Geometry check sheet. Reference: the model listing, model coordinates, mm. A direction names the side the tool comes from. Round coordinates to 2 decimals unless told otherwise and drop trailing zeros. Order: outer loops, then holes, each group sorted by start corner. A loop starts at its lowest first (then second) coordinate and runs counter-clockwise, first axis right, second up.
```python
from build123d import *

# Parameters (mm, degrees)
EXTRUDE_1_DEPTH          = 2
EXTRUDE_1_2_DEPTH        = 2
EXTRUDE_3_DEPTH          = 33.5
EXTRUDE_3_DEPTH_BACK     = 33.5
CUT_EXTRUDE_3_DEPTH      = 154.195952949
CUT_EXTRUDE_3_DEPTH_BACK = 33.5
CUT_EXTRUDE_6_DEPTH      = 154.195952949


with BuildPart() as part:
    # Sketch 1 → Extrude 1 (new body)
    with BuildSketch(Plane(origin=(0, 0, 0), x_dir=(1, 0, 0), z_dir=(0, 1, 0))):
        with BuildLine():
            Line((0, 29), (0, 18))
            ThreePointArc((0, 18), (1.757359313, 13.757359313), (6, 12))
            Line((6, 12), (10, 12))
            Line((10, 12), (10, 10))
            ThreePointArc((10, 10), (12.928932188, 2.928932188), (20, 0))
            Line((20, 0), (90, 0))
            ThreePointArc((90, 0), (97.071067812, 2.928932188), (100, 10))
            Line((100, 10), (100, 12))
            Line((100, 12), (104, 12))
            ThreePointArc((104, 12), (108.242640687, 13.757359313), (110, 18))
            Line((110, 18), (110, 29))
            ThreePointArc((110, 29), (107.656854249, 34.656854249), (102, 37))
            Line((102, 37), (8, 37))
            ThreePointArc((8, 37), (2.343145751, 34.656854249), (0, 29))
        make_face()
        with BuildLine():
            Line((102, 30), (96, 30))
            ThreePointArc((96, 30), (94, 28), (96, 26))
            Line((96, 26), (102, 26))
            ThreePointArc((102, 26), (104, 28), (102, 30))
        make_face(mode=Mode.SUBTRACT)
        with BuildLine():
            Line((8, 26), (14, 26))
            ThreePointArc((14, 26), (16, 28), (14, 30))
            Line((14, 30), (8, 30))
            ThreePointArc((8, 30), (6, 28), (8, 26))
        make_face(mode=Mode.SUBTRACT)
    extrude(amount=EXTRUDE_1_DEPTH)



with BuildPart() as body_2:
    # Sketch 1 → Extrude 1 2 (new body)
    with BuildSketch(Plane(origin=(0, 0, 0), x_dir=(1, 0, 0), z_dir=(0, 1, 0))):
        with BuildLine():
            Line((100, -75), (104, -75))
            ThreePointArc((104, -75), (108.242640687, -76.757359313), (110, -81))
            Line((110, -81), (110, -92))
            ThreePointArc((110, -92), (107.656854249, -97.656854249), (102, -100))
            Line((102, -100), (8, -100))
            ThreePointArc((8, -100), (2.343145751, -97.656854249), (0, -92))
            Line((0, -92), (0, -81))
            ThreePointArc((0, -81), (1.757359313, -76.757359313), (6, -75))
            Line((6, -75), (10, -75))
            Line((10, -75), (10, -73))
            ThreePointArc((10, -73), (12.928932188, -65.928932188), (20, -63))
            Line((20, -63), (90, -63))
            ThreePointArc((90, -63), (97.071067812, -65.928932188), (100, -73))
            Line((100, -73), (100, -75))
        make_face()
        with BuildLine():
            Line((8, -93), (14, -93))
            ThreePointArc((14, -93), (16, -91), (14, -89))
            Line((14, -89), (8, -89))
            ThreePointArc((8, -89), (6, -91), (8, -93))
        make_face(mode=Mode.SUBTRACT)
        with BuildLine():
            Line((102, -89), (96, -89))
            ThreePointArc((96, -89), (94, -91), (96, -93))
            Line((96, -93), (102, -93))
            ThreePointArc((102, -93), (104, -91), (102, -89))
        make_face(mode=Mode.SUBTRACT)
    extrude(amount=EXTRUDE_1_2_DEPTH)


with BuildPart() as part_1:
    add(part.part)

    add(body_2.part)  # Extrude 3 merges body 2
    # Sketch 2 → Extrude 3 (add, two sides: drawn at the far end of the back side and taken through both)
    with BuildSketch(Plane.XY.offset(31.5).offset(-EXTRUDE_3_DEPTH_BACK)):
        Polygon((20, 2), (90, 2), (75.5, 37), (55, 37), (34.5, 37), align=None)
    extrude(amount=EXTRUDE_3_DEPTH + EXTRUDE_3_DEPTH_BACK)

    # Sketch 3 → Cut-Extrude 3 (cut, two sides: drawn at the far end of the back side and taken through both)
    with BuildSketch(Plane(origin=(0, 0, 0), x_dir=(0, 0, -1), z_dir=(1, 0, 0)).offset(-CUT_EXTRUDE_3_DEPTH_BACK)):
        with BuildLine():
            Line((-63, 2), (-63, 1))
            ThreePointArc((-63, 1), (-63.292893219, 0.292893219), (-64, 0))
            Line((-64, 0), (1, 0))
            ThreePointArc((1, 0), (0.292893219, 0.292893219), (0, 1))
            Line((0, 1), (0, 2))
            Line((0, 2), (0, 35))
            Line((0, 35), (-63, 35))
            Line((-63, 35), (-63, 2))
        make_face()
    extrude(amount=CUT_EXTRUDE_3_DEPTH + CUT_EXTRUDE_3_DEPTH_BACK, mode=Mode.SUBTRACT)

    # Sketch 4 → Cut-Extrude 6 (cut, through all)
    with BuildSketch(Plane(origin=(0, 0, 0), x_dir=(1, 0, 0), z_dir=(0, 1, 0))):
        with BuildLine():
            Line((48, -8), (44.5, -8))
            Line((44.5, -8), (44.5, -55))
            Line((44.5, -55), (48, -55))
            Line((48, -55), (48, -58))
            ThreePointArc((48, -58), (50, -60), (52, -58))
            Line((52, -58), (52, -55))
            Line((52, -55), (53.5, -55))
            Line((53.5, -55), (53.5, -58.5))
            ThreePointArc((53.5, -58.5), (55, -60), (56.5, -58.5))
            Line((56.5, -58.5), (56.5, -55))
            Line((56.5, -55), (58, -55))
            Line((58, -55), (58, -58))
            ThreePointArc((58, -58), (60, -60), (62, -58))
            Line((62, -58), (62, -55))
            Line((62, -55), (65.5, -55))
            Line((65.5, -55), (65.5, -8))
            Line((65.5, -8), (62, -8))
            Line((62, -8), (62, -5))
            ThreePointArc((62, -5), (60, -3), (58, -5))
            Line((58, -5), (58, -8))
            Line((58, -8), (56.5, -8))
            Line((56.5, -8), (56.5, -4.5))
            ThreePointArc((56.5, -4.5), (55, -3), (53.5, -4.5))
            Line((53.5, -4.5), (53.5, -8))
            Line((53.5, -8), (52, -8))
            Line((52, -8), (52, -5))
            ThreePointArc((52, -5), (50, -3), (48, -5))
            Line((48, -5), (48, -8))
        make_face()
    extrude(amount=CUT_EXTRUDE_6_DEPTH, mode=Mode.SUBTRACT)


solid = part_1.part
```
(1) Material ranges on line 1 (Z direction, x = 69, y = 8); line 2 (Y direction, x = 74.5, z = 48); line 3 (Y direction, x = 19, z = 78), recorded low to high.
Returned:
line 1: z = -2 to 0, 63 to 65
line 2: y = 35 to 37
line 3: y = 0 to 2
(2) Sectioned sample at C-C, the plane y = 6. Record the cut outline in (x, z).
Returned:
outline: (21.66, -2) - (88.34, -2) - (88.34, 0) - (21.66, 0) - close; (21.66, 63) - (88.34, 63) - (88.34, 65) - (21.66, 65) - close
(3) Sectioned sample at B-B, the plane z = 11. Record the cut outline in (x, y), and give its area (3 significant figures).
Returned:
outline: (33.67, 35) - (44.5, 35) - (44.5, 37) - (34.5, 37) - close; (65.5, 35) - (76.33, 35) - (75.5, 37) - (65.5, 37) - close
area: 41.7 mm2
(4) Sectioned sample at A-A, the plane x = 60. Record the cut outline in (y, z), and give its area (3 significant figures).
Returned:
outline: (0, -37) - (2, -37) - (2, -2) - (37, -2) - (37, 3) - (35, 3) - (35, 0) - (1, 0) arc R1 ccw to (0, -1) - close; (0, 64) arc R1 ccw to (1, 63) - (35, 63) - (35, 60) - (37, 60) - (37, 65) - (2, 65) - (2, 100) - (0, 100) - close
area: 300 mm2
(5) Draft check along Z on faces 1 (the flat face through (56, 0, 82)), 2 (the cylindrical face through (107.719, 0.986, -34.594)), 3 (the cylindrical face through (12.85, 0.99, 66.01)). Enter one of: released by +Z, released by -Z, zero draft, split by the parting line, or undercut.
Returned:
face 1: zero draft
face 2: released by -Z
face 3: undercut
(6) Sectioned sample at D-D, the plane x = 74. Record the cut outline in (y, z), and give its area (3 significant figures).
Returned:
outline: (0, -37) - (2, -37) - (2, -2) - (37, -2) - (37, 65) - (2, 65) - (2, 100) - (0, 100) - (0, 64) arc R1 ccw to (1, 63) - (35, 63) - (35, 0) - (1, 0) arc R1 ccw to (0, -1) - close
area: 414 mm2
(7) Depth check by flat-ended pin: P1, Ø1.6, axis at y = 36, z = 6, coming from the -X side; P2, Ø2, axis at x = 64, y = 36, coming from the -Z side; P3, Ø8, axis at y = 27, z = -3.5, coming from the +X side. Enter the tip coordinate at first touch or a pass-through.
Returned:
P1: stops at x = 33.75
P2: stops at z = -2
P3: stops at x = 81.18
(8) Set-up check for faces 4 (the cylindrical face through (108.196, 0.986, 76.711)), 5 (the flat face through (69, 35, 31)), 6 (the cylindrical face through (1.711, 0.986, -13.804)), 7 (the flat face through (55, 20, -2)): record each of +Z, -Z, +X, -X, +Y, -Y from which the full face is reachable in a straight line by a thin tool's end or side.
Returned:
face 4: +X, +Y, -Y
face 5: +X, -X, -Y
face 6: -X, +Y, -Y
face 7: -Z, +X, -X, +Y
